Design review of the part built by this model. Coordinates are the model's own, in mm. A direction names the side the tool comes from. Round coordinates to 2 decimals unless told otherwise and drop trailing zeros. Order: outer loops, then holes, each group sorted by start corner. A loop starts at its lowest first (then second) coordinate and runs counter-clockwise, first axis right, second up.
from build123d import *

# Parameters (mm, degrees)
SKETCH1_R           = 6.5
BOSS_EXTRUDE1_DEPTH = 9
SKETCH2_R           = 1.1
CUT_EXTRUDE1_DEPTH  = 3
SKETCH3_R           = 1
CUT_EXTRUDE2_DEPTH  = 20
CUT_EXTRUDE3_DEPTH  = 7.5
SKETCH6_W           = 6.8
SKETCH6_H           = 6.8
CUT_EXTRUDE4_DEPTH  = 5
SKETCH7_W           = 2.4
SKETCH7_H           = 2.4
CUT_EXTRUDE5_DEPTH  = 5
FILLET2_R           = 4
SKETCH8_R           = 1
CUT_EXTRUDE6_DEPTH  = 20
SKETCH9_R           = 7.5
CUT_EXTRUDE7_DEPTH  = 0.8
SKETCH11_W          = 5
SKETCH11_H          = 1
BOSS_EXTRUDE2_DEPTH = 5
SKETCH12_W          = 53.006357488
SKETCH12_H          = 54.029399369
SKETCH12_R          = 11
CUT_EXTRUDE9_DEPTH  = 10
FILLET3_R           = 4


with BuildPart() as part:
    # Sketch1 → Boss-Extrude1 (new body)
    with BuildSketch(Plane(origin=(0, 0, 0), x_dir=(1, 0, 0), z_dir=(0, 1, 0))):
        with BuildLine():
            Line((-11, 0), (-11, 22.01))
            ThreePointArc((-11, 22.01), (-7.781103525, 29.781103525), (-0.01, 33))
            Line((-0.01, 33), (0.01, 33))
            ThreePointArc((0.01, 33), (7.781103525, 29.781103525), (11, 22.01))
            Line((11, 22.01), (11, 0))
            ThreePointArc((11, 0), (0, -11), (-11, 0))
        make_face()
        Circle(SKETCH1_R, mode=Mode.SUBTRACT)
    extrude(amount=BOSS_EXTRUDE1_DEPTH)

    # Sketch2 → Cut-Extrude1 (cut)
    with BuildSketch(Plane(origin=(0, 9, 0), x_dir=(1, 0, 0), z_dir=(0, 1, 0))):
        with Locations((-7.15, 5.85)):
            Circle(SKETCH2_R)
        with Locations((-7.15, -5.85)):
            Circle(SKETCH2_R)
        with Locations((7.15, -5.85)):
            Circle(SKETCH2_R)
        with Locations((7.15, 5.85)):
            Circle(SKETCH2_R)
    extrude(amount=-CUT_EXTRUDE1_DEPTH, mode=Mode.SUBTRACT)

    # Sketch3 → Cut-Extrude2 (cut)
    with BuildSketch(Plane(origin=(0, 9, 0), x_dir=(1, 0, 0), z_dir=(0, 1, 0))):
        with Locations((-9, 0)):
            Circle(SKETCH3_R)
        with Locations((9, 0)):
            Circle(SKETCH3_R)
    extrude(amount=-CUT_EXTRUDE2_DEPTH, mode=Mode.SUBTRACT)

    # Sketch4 → Cut-Extrude3 (cut)
    with BuildSketch(Plane.XZ):
        with BuildLine():
            Line((-9, 2.25), (-10.767427734, 2.25))
            Line((-10.767427734, 2.25), (-12, 0))
            Line((-12, 0), (-11, -2.25))
            Line((-11, -2.25), (-9, -2.25))
            ThreePointArc((-9, -2.25), (-6.75, 0), (-9, 2.25))
        make_face()
        with BuildLine():
            Line((12, 0), (10.767427734, 2.25))
            Line((10.767427734, 2.25), (9, 2.25))
            ThreePointArc((9, 2.25), (6.75, 0), (9, -2.25))
            Line((9, -2.25), (11, -2.25))
            Line((11, -2.25), (12, 0))
        make_face()
    extrude(amount=-CUT_EXTRUDE3_DEPTH, mode=Mode.SUBTRACT)

    # Sketch6 → Cut-Extrude4 (cut)
    with BuildSketch(Plane.XZ):
        with Locations((0, -22.01)):
            Rectangle(SKETCH6_W, SKETCH6_H)
    extrude(amount=-CUT_EXTRUDE4_DEPTH, mode=Mode.SUBTRACT)

    # Sketch7 → Cut-Extrude5 (cut)
    with BuildSketch(Plane.XZ.offset(-5)):
        with Locations((2.2, -19.81)):
            Rectangle(SKETCH7_W, SKETCH7_H)
        with Locations((-2.2, -19.81)):
            Rectangle(SKETCH7_W, SKETCH7_H)
        with Locations((2.2, -24.21)):
            Rectangle(SKETCH7_W, SKETCH7_H)
        with Locations((-2.2, -24.21)):
            Rectangle(SKETCH7_W, SKETCH7_H)
    extrude(amount=-CUT_EXTRUDE5_DEPTH, mode=Mode.SUBTRACT)

    # Fillet2
    fillet2_edges = [part.edges().sort_by_distance(p)[0] for p in [
        (0, 0, 11),
    ]]
    fillet(fillet2_edges, radius=FILLET2_R)

    # Sketch8 → Cut-Extrude6 (cut)
    with BuildSketch(Plane.XZ):
        with Locations((-9, -22.01)):
            Circle(SKETCH8_R)
        with Locations((9, -22.01)):
            Circle(SKETCH8_R)
    extrude(amount=-CUT_EXTRUDE6_DEPTH, mode=Mode.SUBTRACT)

    # Sketch9 → Cut-Extrude7 (cut)
    with BuildSketch(Plane(origin=(0, 9, 0), x_dir=(1, 0, 0), z_dir=(0, 1, 0))):
        Circle(SKETCH9_R)
    extrude(amount=-CUT_EXTRUDE7_DEPTH, mode=Mode.SUBTRACT)

    # Sketch11 → Boss-Extrude2 (add)
    with BuildSketch(Plane.ZY.offset(-3.4)):
        with Locations((-14.185057965, 8.5)):
            Rectangle(SKETCH11_W, SKETCH11_H)
    extrude(amount=BOSS_EXTRUDE2_DEPTH)

    # Sketch12 → Cut-Extrude9 (cut)
    with BuildSketch(Plane.XZ):
        with Locations((2.65351488, -12.086981999)):
            Rectangle(SKETCH12_W, SKETCH12_H)
        Circle(SKETCH12_R, mode=Mode.SUBTRACT)
    extrude(amount=-CUT_EXTRUDE9_DEPTH, mode=Mode.SUBTRACT)

    # Fillet3
    fillet3_edges = [part.edges().sort_by_distance(p)[0] for p in [
        (0, 0, -11),
    ]]
    fillet(fillet3_edges, radius=FILLET3_R)


solid = part.part
1) To check wall thickness, follow line 1 along Z through (x, y) = (0, 8.4); line 2 along Z through (x, y) = (-7.15, 8); line 3 along X through (y, z) = (8.5, 5.75). State the ranges of each line that lie inside material, in increasing order.
Results:
line 1: z = -11 to -7.5, 7.5 to 11
line 2: z = -8.36 to -6.95, -4.75 to 4.75, 6.95 to 8.36
line 3: x = -9.38 to -8.25, -6.05 to -4.82, 4.82 to 6.05, 8.25 to 9.38
2) Take a section at D-D on y = 1.75. Give the boundary of the cut face in (x, z).
Results:
outline: (-10.06, -2.25) arc R10.31 ccw to (10.06, -2.25) - (9, -2.25) arc R2.25 cw to (9, 2.25) - (10.06, 2.25) arc R10.31 ccw to (-10.06, 2.25) - (-9, 2.25) arc R2.25 cw to (-9, -2.25) - close; hole circle Ø13 at (0, 0)
3) The part is to be moulded in two halves that separate along Z. For faces 5 (the face through (2.6, 9, 7.2)), 6 (the face through (10.161, 6.465, -4.213)), 7 (the face through (-7, 6, -6)), say which applies: released by +Z, released by -Z, zero draft, split by the parting line, or undercut.
Results:
face 5: zero draft
face 6: split by the parting line
face 7: undercut
4) Take a section at A-A on z = 0. Give the boundary of the cut face in (x, y).
Results:
outline: (-11, 7.5) - (-10, 7.5) - (-10, 9) - (-11, 9) - close; (-8, 7.5) - (-6.75, 7.5) - (-6.75, 0) - (-6.5, 0) - (-6.5, 8.2) - (-7.5, 8.2) - (-7.5, 9) - (-8, 9) - close; (6.5, 0) - (6.75, 0) - (6.75, 7.5) - (8, 7.5) - (8, 9) - (7.5, 9) - (7.5, 8.2) - (6.5, 8.2) - close; (10, 7.5) - (11, 7.5) - (11, 9) - (10, 9) - close
5) For faces 1 (the face through (-6.75, 3.7, -0.05)), 2 (the face through (10.3, 7.5, 0)), 3 (the face through (-9.8, 8.3, 0.6)), 4 (the face through (-6.134, 7.521, 6.271)), list the 3-axis set-ups (+Z, -Z, +X, -X, +Y, -Y) from which the entire face can be reached by the end or side of a thin tool; tool diameter is ignored.
Results:
face 1: -X, -Y
face 2: +X, -Y
face 3: +Y, -Y
face 4: +Y
6) Take a section at B-B on x = 0. Give the boundary of the cut face in (y, z).
Results:
outline: (0, -7) arc R4 ccw to (4, -11) - (9, -11) - (9, -7.5) - (8.2, -7.5) - (8.2, -6.5) - (0, -6.5) - close; (0, 6.5) - (8.2, 6.5) - (8.2, 7.5) - (9, 7.5) - (9, 11) - (4, 11) arc R4 ccw to (0, 7) - close
7) Take a section at C-C on y = 7. Give the boundary of the cut face in (x, z).
Results:
outline: (-10.77, -2.25) arc R11 ccw to (10.77, -2.25) - (9, -2.25) arc R2.25 cw to (9, 2.25) - (10.77, 2.25) arc R11 ccw to (-10.77, 2.25) - (-9, 2.25) arc R2.25 cw to (-9, -2.25) - close; hole circle Ø2.2 at (-7.15, -5.85); hole circle Ø2.2 at (-7.15, 5.85); hole circle Ø13 at (0, 0); hole circle Ø2.2 at (7.15, -5.85); hole circle Ø2.2 at (7.15, 5.85)
8) Clearance check with flat-ended pins moving along their axes: P1, Ø3, axis at x = -7, y = 3, coming from the +Z side; P2, Ø4.5, axis at x = 9, z = 0.5, coming from the -Y side; P3, Ø1.9, axis at x = 10, y = 3, coming from the -Z side; P4, Ø1.3, axis at x = 7.15, z = -5.85, coming from the -Y side. State where each tip first meets the part, or that it passes through.
Results:
P1: stops at z = 9.44
P2: stops at y = 0
P3: stops at z = -6.08
P4: stops at y = 0.33
